Print and shaded views of the part. All mm, measured from the part's lowest x, y and z. A direction names the side the tool comes from. Round coordinates to 2 decimals unless told otherwise and drop trailing zeros. Loops run counter-clockwise (first coordinate to the right, second up) from the corner with the lowest first, then second, coordinate; pieces in that order, holes last. Notation, with made-up numbers: (68.5, 59) - (84.5, 59) arc R7 ccw to (84.5, 64) - close; hole circle Ø10 at (59.5, 64.25). An arc over 180 degrees is marked (long way). Use one line per item in the form item = value.
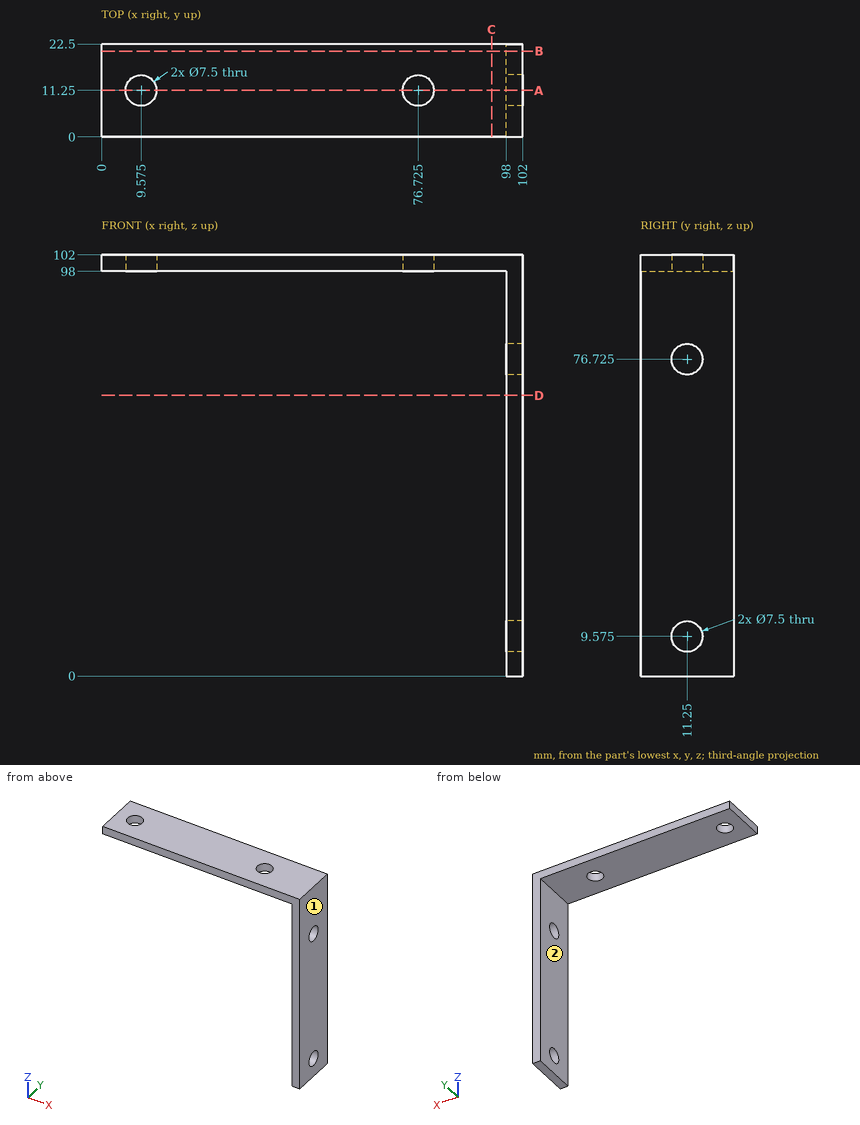
1. Cut at D-D, the plane z = 68. Give the cut face in (x, y), plus the area to 3 significant figures.
Geometry check:
outline = (98, 0) - (102, 0) - (102, 22.5) - (98, 22.5) - close
area = 90.0 mm^2
2. Tool access for the marked faces 1 and 2: list every direction of +Z, -Z, +X, -X, +Y, -Y with a clear straight run to the whole face (end or side of a thin tool).
Geometry check:
face_1 = +Z, -Z, +X, +Y, -Y
face_2 = -Z, -X, +Y, -Y
3. Cut at B-B, the plane y = 20.75. Give the cut face in (x, z).
Geometry check:
outline = (0, 98) - (98, 98) - (98, 0) - (102, 0) - (102, 102) - (0, 102) - close
4. Cut at A-A, the plane y = 11.25. Give the cut face in (x, z) (3 decimals), plus the area to 3 significant figures.
Geometry check:
outline = (0, 98) - (5.825, 98) - (5.825, 102) - (0, 102) - close; (13.325, 98) - (72.975, 98) - (72.975, 102) - (13.325, 102) - close; (80.475, 98) - (98, 98) - (98, 80.475) - (102, 80.475) - (102, 102) - (80.475, 102) - close; (98, 0) - (102, 0) - (102, 5.825) - (98, 5.825) - close; (98, 13.325) - (102, 13.325) - (102, 72.975) - (98, 72.975) - close
area = 680 mm^2
5. Flat gauge pins, fed straight in: pin 1 (7 mm diameter, centred on y = 12.5, z = 72.5, fed in from -X); pin 2 (10 mm diameter, centred on x = 67.5, y = 16.5, fed in from -Z); pin 3 (6 mm diameter, centred on x = 76.725, y = 11.25, fed in from +Z). Where does each tip first touch, or does it go through?
Geometry check:
pin_1 = 98
pin_2 = 98
pin_3 = through
6. Wall check: probe 1 along Z at (x, y) = (100, 11.25) (3 decimals); probe 2 along Z at (x, y) = (7.5, 17.25). Give the ranges that are in metal, low to high.
Geometry check:
probe_1 = 0 to 5.825, 13.325 to 72.975, 80.475 to 102
probe_2 = 98 to 102
7. Cut at C-C, the plane x = 94.5. Give the cut face in (y, z), plus the area to 3 significant figures.
Geometry check:
outline = (0, 98) - (22.5, 98) - (22.5, 102) - (0, 102) - close
area = 90.0 mm^2
